Build history of the part. All positions in model axes, mm. A direction names the side the tool comes from. Give positions to 0.01 mm unless a question says otherwise; leave off trailing zeros. Order: outer loops, then holes, each group sorted by start corner. A loop starts at its lowest first (then second) coordinate and runs counter-clockwise, first axis right, second up. Notation, with made-up numbers: (12, -19) -> (70, -19) arc R6 ccw to (70, -14) -> close; hole circle Ø11 at (36, 65). An arc over 180 degrees is marked (long way). One line per item, written item: value. Start each with the question number.
(1) Probe line 1 (Y direction, x = -125.5, z = -6.5); line 2 (X direction, y = 28, z = -11); line 3 (Z direction, x = -19, y = 50.5). List the from-to ranges inside material, lowest first.
(2) Saw through at B-B on y = -21.3. Give the cut face in (x, z).
(3) Saw through at C-C on x = -85. Give the cut face in (y, z), plus the area to 3 significant figures.
(4) Pin check, flat tips, straight feed: pin 1 (5 mm diameter, centred on x = -109.49, y = 3.64, fed in from +Z); pin 2 (3.5 mm diameter, centred on y = -21.3, z = -29.13, fed in from -X). Stop position of each tip, or through.
(5) Which spindle directions (+Z, -Z, +X, -X, +Y, -Y) get a long thin tool onto all of the face, cutting with end or side? Do faces 4 (the cylindrical face through (-144.7, -22.1, -27.3)), 5 (the flat face through (44, 35.735, -30)), 6 (the flat face through (27.105, -44, -17)), 7 (the flat face through (-49, 16, -43.297)). Say none if no direction does.
(6) Two-plate mould, pull along Y, no slides. Class faces 1 (the flat face through (44, 13, -24.714)), 2 (the flat face through (-147.124, 14, -18)), 3 (the flat face through (-49, -46.3, -18)): +Y half, -Y half, draft (parallel to the pull), parting line (faces both ways), or undercut.
(7) Saw through at A-A on x = -31.5. Give the cut face in (y, z).
```python
from build123d import *

# Parameters (mm, degrees)
SCHIZZO2_W                   = 194.047297703
SCHIZZO2_H                   = 123.066886556
SCHIZZO2_W_2                 = 184.047297703
SCHIZZO2_H_2                 = 113.066886556
ESTRUSIONE_SOTTILE1_DEPTH    = 45
SCHIZZO3_W                   = 194.047297703
SCHIZZO3_H                   = 123.066886556
ESTRUSIONE_ESTRUSIONE1_DEPTH = 5
SCHIZZO4_R                   = 2
TAGLIO_ESTRUSIONE1_DEPTH     = 5
SMUSSO1_SIZE                 = 1.5
SMUSSO2_SIZE                 = 1.5
SMUSSO3_SIZE                 = 1.5
SMUSSO4_SIZE                 = 1.5
SCHIZZO5_W                   = 7.767621353
SCHIZZO5_H                   = 19.92122066
SCHIZZO5_W_2                 = 7.310576499
SCHIZZO5_H_2                 = 13.99005078
SCHIZZO5_W_3                 = 12.838114045
SCHIZZO5_H_3                 = 10.076749863
SCHIZZO5_W_4                 = 11.950153196
SCHIZZO5_H_4                 = 31.877712984
TAGLIO_ESTRUSIONE2_DEPTH     = 5
SCHIZZO6_W                   = 17.563316518
SCHIZZO6_H                   = 14.837974299
SCHIZZO6_W_2                 = 14.53926904
SCHIZZO6_H_2                 = 16.284185158
SCHIZZO6_W_3                 = 14.178791295
TAGLIO_ESTRUSIONE3_DEPTH     = 5
SMUSSO5_SIZE                 = 1.5
SMUSSO6_SIZE                 = 1.5
SCHIZZO7_R                   = 2
TAGLIO_ESTRUSIONE4_DEPTH     = 5
TAGLIO_ESTRUSIONE5_REACH     = 215.125
SCHIZZO8_R                   = 1.25
TAGLIO_ESTRUSIONE6_REACH     = 198.636
SCHIZZO9_R                   = 1.25
SCHIZZO10_R                  = 1.5
TAGLIO_ESTRUSIONE7_DEPTH     = 10
SCHIZZO11_R                  = 4
TAGLIO_ESTRUSIONE8_DEPTH     = 10


with BuildPart() as part:
    # Schizzo2 → Estrusione-Sottile1 (new body)
    with BuildSketch(Plane.XY.offset(6.703232706)):
        with Locations((-50.100447002, 15.233443278)):
            Rectangle(SCHIZZO2_W, SCHIZZO2_H)
        with Locations((-50.100447002, 15.233443278)):
            Rectangle(SCHIZZO2_W_2, SCHIZZO2_H_2, mode=Mode.SUBTRACT)
    extrude(amount=-ESTRUSIONE_SOTTILE1_DEPTH)

    # Schizzo3 → Estrusione-Estrusione1 (add)
    with BuildSketch(Plane(origin=(0, 0, -38.296767294), x_dir=(-1, 0, 0), z_dir=(0, 0, -1))):
        with Locations((50.100447002, 15.233443278)):
            Rectangle(SCHIZZO3_W, SCHIZZO3_H)
    extrude(amount=ESTRUSIONE_ESTRUSIONE1_DEPTH)

    # Schizzo4 → Taglio-Estrusione1 (cut)
    with BuildSketch(Plane.XY.offset(-38.296767294)):
        with Locations((-40.051479808, 38.040961433)):
            Circle(SCHIZZO4_R)
        with Locations((-40.062752428, -30.759038567)):
            Circle(SCHIZZO4_R)
        with Locations((31.337247572, 38.040961433)):
            Circle(SCHIZZO4_R)
        with Locations((31.337247572, -30.759038567)):
            Circle(SCHIZZO4_R)
    extrude(amount=-TAGLIO_ESTRUSIONE1_DEPTH, mode=Mode.SUBTRACT)

    # Smusso1
    smusso1_edges = [part.edges().sort_by_distance(p)[0] for p in [
        (-42.051479808, 38.040961433, -43.296767294),
    ]]
    chamfer(smusso1_edges, length=SMUSSO1_SIZE)

    # Smusso2
    smusso2_edges = [part.edges().sort_by_distance(p)[0] for p in [
        (29.337247572, 38.040961433, -43.296767294),
    ]]
    chamfer(smusso2_edges, length=SMUSSO2_SIZE)

    # Smusso3
    smusso3_edges = [part.edges().sort_by_distance(p)[0] for p in [
        (29.337247572, -30.759038567, -43.296767294),
    ]]
    chamfer(smusso3_edges, length=SMUSSO3_SIZE)

    # Smusso4
    smusso4_edges = [part.edges().sort_by_distance(p)[0] for p in [
        (-42.062752428, -30.759038567, -43.296767294),
    ]]
    chamfer(smusso4_edges, length=SMUSSO4_SIZE)

    # Schizzo5 → Taglio-Estrusione2 (cut)
    with BuildSketch(Plane(origin=(46.92320185, 0, 0), x_dir=(0, 0, -1), z_dir=(1, 0, 0))):
        with Locations((28.867264407, 25.774079034)):
            Rectangle(SCHIZZO5_W, SCHIZZO5_H)
        with Locations((21.058264637, 12.710451031)):
            Rectangle(SCHIZZO5_W_2, SCHIZZO5_H_2)
        with Locations((18.294495864, 0.187888095)):
            Rectangle(SCHIZZO5_W_3, SCHIZZO5_H_3)
        with Locations((18.13726933, -25.361143508)):
            Rectangle(SCHIZZO5_W_4, SCHIZZO5_H_4)
    extrude(amount=-TAGLIO_ESTRUSIONE2_DEPTH, mode=Mode.SUBTRACT)

    # Schizzo6 → Taglio-Estrusione3 (cut)
    with BuildSketch(Plane.XZ.offset(46.3)):
        with Locations((18.323185023, -16.793891295)):
            Rectangle(SCHIZZO6_W, SCHIZZO6_H)
        with Locations((-6.016266439, -16.070785866)):
            Rectangle(SCHIZZO6_W_2, SCHIZZO6_H_2)
        with Locations((-28.245727369, -16.070785866)):
            Rectangle(SCHIZZO6_W_3, SCHIZZO6_H_2)
    extrude(amount=-TAGLIO_ESTRUSIONE3_DEPTH, mode=Mode.SUBTRACT)

    # Smusso5
    smusso5_edges = [part.edges().sort_by_distance(p)[0] for p in [
        (-35.335123016, -46.3, -16.070785866),
        (-28.245727368, -46.3, -24.212878445),
        (-21.156331721, -46.3, -16.070785866),
        (-28.245727368, -46.3, -7.928693287),
    ]]
    chamfer(smusso5_edges, length=SMUSSO5_SIZE)

    # Smusso6
    smusso6_edges = [part.edges().sort_by_distance(p)[0] for p in [
        (46.92320185, 25.774079034, -32.751075083),
    ]]
    chamfer(smusso6_edges, length=SMUSSO6_SIZE)

    # Schizzo7 → Taglio-Estrusione4 (cut)
    with BuildSketch(Plane.ZY.offset(147.124095853)):
        with Locations((-29.134697753, 51.766886556)):
            Circle(SCHIZZO7_R)
        with Locations((-29.134697753, 15.233443278)):
            Circle(SCHIZZO7_R)
        with Locations((-29.134697753, -21.3)):
            Circle(SCHIZZO7_R)
    extrude(amount=-TAGLIO_ESTRUSIONE4_DEPTH, mode=Mode.SUBTRACT)

    # Schizzo8 → Taglio-Estrusione5 (cut, up to next)
    with BuildSketch(Plane.ZY.offset(147.124095853), mode=Mode.PRIVATE) as taglio_estrusione5_sk1:
        with Locations((4.203232706, 15.309766732)):
            Circle(SCHIZZO8_R)
    taglio_estrusione5_tool1 = extrude(taglio_estrusione5_sk1.sketch, amount=-TAGLIO_ESTRUSIONE5_REACH, mode=Mode.PRIVATE) & part.part
    add(taglio_estrusione5_tool1.solids().sort_by_distance((-147.124096, 15.309767, 4.203233))[0], mode=Mode.SUBTRACT)
    add(taglio_estrusione5_tool1.solids().sort_by_distance((-147.124096, 15.309767, 4.203233))[1], mode=Mode.SUBTRACT)

    # Schizzo9 → Taglio-Estrusione6 (cut, up to next)
    with BuildSketch(Plane.XZ.offset(46.3), mode=Mode.PRIVATE) as taglio_estrusione6_sk1:
        with Locations(Location((-50.100447002, 4.203232706, 0), (0, 0, 270))):
            Circle(SCHIZZO9_R)
    taglio_estrusione6_tool1 = extrude(taglio_estrusione6_sk1.sketch, amount=-TAGLIO_ESTRUSIONE6_REACH, mode=Mode.PRIVATE) & part.part
    add(taglio_estrusione6_tool1.solids().sort_by_distance((-50.100447, -46.3, 4.203233))[0], mode=Mode.SUBTRACT)
    add(taglio_estrusione6_tool1.solids().sort_by_distance((-50.100447, -46.3, 4.203233))[1], mode=Mode.SUBTRACT)

    # Schizzo10 → Taglio-Estrusione7 (cut)
    with BuildSketch(Plane(origin=(0, 0, -43.296767294), x_dir=(-1, 0, 0), z_dir=(0, 0, -1))):
        with Locations((79.486260937, 38.040961433)):
            Circle(SCHIZZO10_R)
        with Locations((109.486260937, 38.040961433)):
            Circle(SCHIZZO10_R)
        with Locations((109.486260937, -30.759038567)):
            Circle(SCHIZZO10_R)
        with Locations((79.486260937, -30.759038567)):
            Circle(SCHIZZO10_R)
        with Locations((109.486260937, 3.640961433)):
            Circle(SCHIZZO10_R)
        with Locations((79.486260937, 3.640961433)):
            Circle(SCHIZZO10_R)
    extrude(amount=-TAGLIO_ESTRUSIONE7_DEPTH, mode=Mode.SUBTRACT)

    # Schizzo11 → Taglio-Estrusione8 (cut)
    with BuildSketch(Plane.XZ.offset(46.3)):
        with Locations(Location((-129.330552929, -18.296767294, 0), (0, 0, 270))):
            Circle(SCHIZZO11_R)
    extrude(amount=-TAGLIO_ESTRUSIONE8_DEPTH, mode=Mode.SUBTRACT)


solid = part.part
```
Results below:
1. line 1: y = -46.3 to -41.3, 71.77 to 76.77
1. line 2: x = -147.12 to -142.12, 41.92 to 46.92
1. line 3: z = -43.3 to -38.3
2. outline: (-147.12, -43.3) -> (46.92, -43.3) -> (46.92, -24.11) -> (41.92, -24.11) -> (41.92, -38.3) -> (-142.12, -38.3) -> (-142.12, -31.13) -> (-147.12, -31.13) -> close; (-147.12, -27.13) -> (-142.12, -27.13) -> (-142.12, 6.7) -> (-147.12, 6.7) -> close; (41.92, -12.16) -> (46.92, -12.16) -> (46.92, 6.7) -> (41.92, 6.7) -> close
3. outline: (-46.3, -43.3) -> (76.77, -43.3) -> (76.77, 6.7) -> (71.77, 6.7) -> (71.77, -38.3) -> (-41.3, -38.3) -> (-41.3, 6.7) -> (-46.3, 6.7) -> close
3. area: 1,070 mm²
4. pin 1: stops at z = -38.3
4. pin 2: stops at x = 41.92
5. face 4: -X
5. face 5: +X
5. face 6: -Y
5. face 7: -Z, +X, -X, +Y, -Y
6. face 1: undercut
6. face 2: draft
6. face 3: -Y half
7. outline: (-46.3, -43.3) -> (76.77, -43.3) -> (76.77, 6.7) -> (71.77, 6.7) -> (71.77, -38.3) -> (-41.3, -38.3) -> (-41.3, -24.21) -> (-44.8, -24.21) -> (-46.3, -25.71) -> close; (-46.3, -6.43) -> (-44.8, -7.93) -> (-41.3, -7.93) -> (-41.3, 6.7) -> (-46.3, 6.7) -> close
